CAD build for the part. Positions are in the model's coordinates, mm. A direction names the side the tool comes from. Give positions to 0.01 mm unless a question says otherwise; leave off trailing zeros. Write each loop counter-clockwise with the first axis right and the second up, starting at its lowest first coordinate (ties: lowest second). Pieces come first, ordered by that corner, then holes. Notation, with made-up numbers: (23.25, 34.25) - (64.25, 34.25) arc R32 cw to (64.25, 69.25) - close; hole circle Ø6 at (66, 21.5). An arc over 180 degrees is marked (long way). Put each result on its own line as item: value. Start each with the question number.
1. Cut at C-C on z = -1.9. List the corners of the cut face in (x, y).
2. Cut at A-A on z = -8.5. List the corners of the cut face in (x, y).
3. Wall check: line 1 (X direction, y = 0.15, z = -8.5); line 2 (X direction, y = -1.5, z = -1.9); line 3 (X direction, y = 1.5, z = -1). Give the ranges that are in metal, low to high.
4. Cut at D-D on x = -4. List the corners of the cut face in (y, z).
5. Tool access for faces 1 (the flat face through (0.8, 0.03, 6.48)), 2 (the flat face through (8, -0.25, -7)), 3 (the flat face through (-1, 0.25, -7)): list every direction of +Z, -Z, +X, -X, +Y, -Y with a clear straight run to the whole face (end or side of a thin tool).
6. Drop flat-ended pins along their axis: pin 1 (2.5 mm diameter, centred on x = -8, z = -8.5, fed in from -Y); pin 2 (2.5 mm diameter, centred on x = 8, z = -7, fed in from +Y); pin 3 (1.5 mm diameter, centred on x = -2, y = 2.5, fed in from +Z). Give the stop position or say it passes through.
7. Mould opens along X. For faces 4 (the cylindrical face through (-1.53, 0.004, -9.294)), 5 (the flat face through (-1, -0.25, -7)), 6 (the flat face through (10, 0, 0)) say: +X half, -X half, draft (parallel to the pull), parting line (faces both ways), or undercut.
8. Cut at B-B on y = 0.5. List the corners of the cut face in (x, z), and give its area (3 significant figures).
from build123d import *

# Parameters (mm, degrees)
SKETCH1_W           = 20
SKETCH1_H           = 10
BOSS_EXTRUDE1_DEPTH = 3.1
BOSS_EXTRUDE3_DEPTH = 2
SKETCH4_W           = 3.2
SKETCH4_H           = 0.5
BOSS_EXTRUDE4_DEPTH = 5
SKETCH7_R           = 1
CUT_EXTRUDE1_DEPTH  = 5
SKETCH8_R           = 1.25
CUT_EXTRUDE2_DEPTH  = 16.473248494


with BuildPart() as part:
    # Sketch1 → Boss-Extrude1 (new, symmetric)
    with BuildSketch(Plane(origin=(0, 0, 0), x_dir=(1, 0, 0), z_dir=(0, 1, 0))):
        Rectangle(SKETCH1_W, SKETCH1_H)
    extrude(amount=BOSS_EXTRUDE1_DEPTH, both=True)

    # Sketch3 → Boss-Extrude3 (add, symmetric)
    with BuildSketch(Plane(origin=(0, 0, 0), x_dir=(1, 0, 0), z_dir=(0, 1, 0))):
        Polygon((-8.139274181, -5), (10, -8), (10.048951137, -7.704020632), (-6.300706076, -5), align=None)
    extrude(amount=BOSS_EXTRUDE3_DEPTH, both=True)

    # Sketch4 → Boss-Extrude4 (add)
    with BuildSketch(Plane(origin=(0, 0, -5), x_dir=(-1, 0, 0), z_dir=(0, 0, -1))):
        with Locations((-7.5, 0)):
            Rectangle(SKETCH4_W, SKETCH4_H)
        with Locations((0.921991111, 0)):
            Rectangle(SKETCH4_W, SKETCH4_H)
        with Locations((8, 0)):
            Rectangle(SKETCH4_W, SKETCH4_H)
    extrude(amount=BOSS_EXTRUDE4_DEPTH)

    # Sketch7 → Cut-Extrude1 (cut)
    with BuildSketch(Plane(origin=(0, 0.25, 0), x_dir=(1, 0, 0), z_dir=(0, 1, 0))):
        with Locations(Location((-8, 8.5, 0), (0, 0, 270))):
            Circle(SKETCH7_R)
        with Locations(Location((-0.921991111, 8.5, 0), (0, 0, 270))):
            Circle(SKETCH7_R)
        with Locations(Location((7.5, 8.5, 0), (0, 0, 270))):
            Circle(SKETCH7_R)
    extrude(amount=-CUT_EXTRUDE1_DEPTH, mode=Mode.SUBTRACT)

    # Sketch8 → Cut-Extrude2 (cut, through all)
    with BuildSketch(Plane(origin=(0, 3.1, 0), x_dir=(1, 0, 0), z_dir=(0, 1, 0))):
        with Locations(Location((-4.75, 1.9, 0), (0, 0, 270))):
            Circle(SKETCH8_R)
        with Locations(Location((4.75, 1.9, 0), (0, 0, 270))):
            Circle(SKETCH8_R)
    extrude(amount=-CUT_EXTRUDE2_DEPTH, mode=Mode.SUBTRACT)


solid = part.part
Report:
1. outline: (-10, -3.1) - (-6, -3.1) - (-6, 3.1) - (-10, 3.1) - close; (-3.5, -3.1) - (3.5, -3.1) - (3.5, 3.1) - (-3.5, 3.1) - close; (6, -3.1) - (10, -3.1) - (10, 3.1) - (6, 3.1) - close
2. outline: (-9.6, -0.25) - (-9, -0.25) - (-9, 0.25) - (-9.6, 0.25) - close; (-7, -0.25) - (-6.4, -0.25) - (-6.4, 0.25) - (-7, 0.25) - close; (-2.52, -0.25) - (-1.92, -0.25) - (-1.92, 0.25) - (-2.52, 0.25) - close; (0.08, -0.25) - (0.68, -0.25) - (0.68, 0.25) - (0.08, 0.25) - close; (5.9, -0.25) - (6.5, -0.25) - (6.5, 0.25) - (5.9, 0.25) - close; (8.5, -0.25) - (9.1, -0.25) - (9.1, 0.25) - (8.5, 0.25) - close
3. line 1: x = -9.6 to -9, -7 to -6.4, -2.52 to -1.92, 0.08 to 0.68, 5.9 to 6.5, 8.5 to 9.1
3. line 2: x = -10 to -6, -3.5 to 3.5, 6 to 10
3. line 3: x = -10 to -5.62, -3.88 to 3.88, 5.62 to 10
4. outline: (-3.1, -5) - (3.1, -5) - (3.1, -2.9) - (-3.1, -2.9) - close; (-3.1, -0.9) - (3.1, -0.9) - (3.1, 5) - (-3.1, 5) - close; (-2, 5.38) - (2, 5.38) - (2, 5.68) - (-2, 5.68) - close
5. face 1: +Z, -X, +Y, -Y
5. face 2: -Z, +X, -X, -Y
5. face 3: -Z, +X, -X, +Y
6. pin 1: stops at y = -0.25
6. pin 2: stops at y = 0.25
6. pin 3: stops at z = 6.11
7. face 4: undercut
7. face 5: draft
7. face 6: +X half
8. outline: (-10, -5) - (10, -5) - (10, 5) - (-6.3, 5) - (10.05, 7.7) - (10, 8) - (-8.14, 5) - (-10, 5) - close; hole circle Ø2.5 at (-4.75, -1.9); hole circle Ø2.5 at (4.75, -1.9)
8. area: 195 mm²
